Part print with two shaded views. Sizes in mm from the minimum x, y, z corner. Give positions to 0.01 mm unless a question says otherwise; leave off trailing zeros. Order: outer loops, then holes, each group sorted by start corner. A loop starts at its lowest first (then second) coordinate and runs counter-clockwise, first axis right, second up.
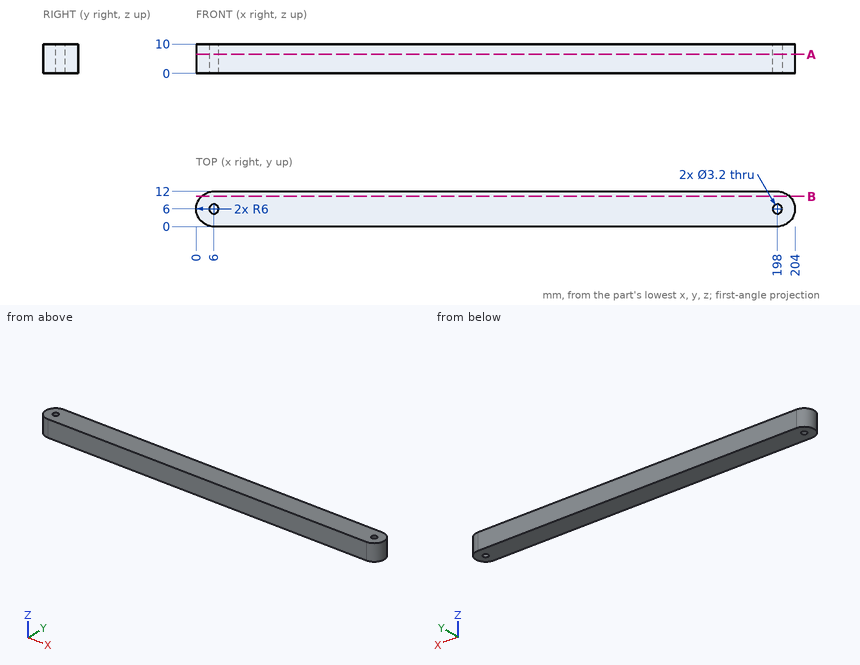
1. Saw through at A-A on z = 6.5. Give the cut face in (x, y), plus the area to 3 significant figures.
2. Pin check, flat tips, straight feed: P1, Ø5, axis at x = 124, y = 3.5, coming from the -Z side; P2, Ø5, axis at y = 1.5, z = 7.5, coming from the +X side; P3, Ø1, axis at y = 3.5, z = 5.5, coming from the -X side; P4, Ø2.5, axis at x = 6, y = 6, coming from the -Z side. Stop position of each tip, or through.
3. Wall check: line 1 (X direction, y = 6.25, z = 1.5); line 2 (Y direction, x = 198, z = 5); line 3 (X direction, y = 8, z = 6). Give the ranges that are in metal, low to high.
4. Saw through at B-B on y = 10.25. Give the cut face in (x, z).
Reported:
1. outline: (6, 0) - (198, 0) arc R6 ccw to (198, 12) - (6, 12) arc R6 ccw to start; hole circle Ø3.2 at (6, 6); hole circle Ø3.2 at (198, 6)
1. area: 2,400 mm2
2. P1: stops at z = 0
2. P2: stops at x = 203.66
2. P3: stops at x = 0.34
2. P4: passes through
3. line 1: x = 0.01 to 4.42, 7.58 to 196.42, 199.58 to 203.99
3. line 2: y = 0 to 4.4, 7.6 to 12
3. line 3: x = 0.34 to 203.66
4. outline: (1.76, 0) - (202.24, 0) - (202.24, 10) - (1.76, 10) - close
